```python
from build123d import *

# Parameters (mm, degrees)
SKETCH1_W           = 1700
SKETCH1_H           = 500
BOSS_EXTRUDE1_DEPTH = 5
SKETCH2_W           = 20
SKETCH2_H           = 20
BOSS_EXTRUDE2_DEPTH = 695
SKETCH3_W           = 900
SKETCH3_H           = 500
BOSS_EXTRUDE3_DEPTH = 30
SKETCH4_W           = 170
SKETCH4_H           = 500
CUT_EXTRUDE1_DEPTH  = 30


with BuildPart() as part:
    # Sketch1 → Boss-Extrude1 (new body)
    with BuildSketch(Plane(origin=(0, 0, 0), x_dir=(1, 0, 0), z_dir=(0, 1, 0))):
        with Locations((850, 250)):
            Rectangle(SKETCH1_W, SKETCH1_H)
    extrude(amount=BOSS_EXTRUDE1_DEPTH)

    # Sketch2 → Boss-Extrude2 (add)
    with BuildSketch(Plane(origin=(0, 5, 0), x_dir=(1, 0, 0), z_dir=(0, 1, 0))):
        with Locations((10, 490)):
            Rectangle(SKETCH2_W, SKETCH2_H)
        with Locations((10, 10)):
            Rectangle(SKETCH2_W, SKETCH2_H)
        with Locations((1690, 10)):
            Rectangle(SKETCH2_W, SKETCH2_H)
        with Locations((1690, 490)):
            Rectangle(SKETCH2_W, SKETCH2_H)
    extrude(amount=BOSS_EXTRUDE2_DEPTH)

    # Sketch3 → Boss-Extrude3 (add)
    with BuildSketch(Plane.XZ):
        with Locations((850, -250)):
            Rectangle(SKETCH3_W, SKETCH3_H)
    extrude(amount=BOSS_EXTRUDE3_DEPTH)

    # Sketch4 → Cut-Extrude1 (cut)
    with BuildSketch(Plane.XZ.offset(30)):
        with Locations((550, -250)):
            Rectangle(SKETCH4_W, SKETCH4_H)
        with Locations((850, -250)):
            Rectangle(SKETCH4_W, SKETCH4_H)
        with Locations((1150, -250)):
            Rectangle(SKETCH4_W, SKETCH4_H)
    extrude(amount=-CUT_EXTRUDE1_DEPTH, mode=Mode.SUBTRACT)


solid = part.part
```
Input: part model. Units: mm. Frame: model coordinates. A direction names the side the tool comes from. Coordinates: 2 decimals unless noted, no trailing zeros. Loops run counter-clockwise (first coordinate to the right, second up) from the corner with the lowest first, then second, coordinate; pieces in that order, holes last. Notation, with made-up numbers: (-36.5, 31.25) - (12.5, 31.25) arc R27 ccw to (12.5, 69.25) - close; hole circle Ø7 at (1.25, 87.5). An arc over 180 degrees is marked (long way). Answer in a Markdown table with one row per item.
(1) Material intervals for L1, parallel to Y at x = 838, z = -229.5; L2, parallel to Y at x = 637, z = -323.5, sorted ascending. Write a range as from..to.
Model answer:
| item | result |
|---|---|
| L1 | y = 0..5 |
| L2 | y = -30..5 |
(2) Mould query, pull axis X, two halves, no side actions, for faces 4 (the face through (699, -30, -246)), 5 (the face through (0, 348, -490)), 6 (the face through (549, 0, -246)). Classes: pulls with the +X half, pulls with the -X half, needs draft (parallel to the pull), parting line crosses it, or undercut.
Model answer:
| item | result |
|---|---|
| face 4 | needs draft |
| face 5 | pulls with the -X half |
| face 6 | undercut |
(3) Set-up query: faces 1 (the face through (1497, 0, -254)), 2 (the face through (465, -15, -253)), 3 (the face through (400, -15, -253)). Return all of +Z, -Z, +X, -X, +Y, -Y with unobstructed straight access to the full face (end or side cutting, diameter ignored); none if empty.
Model answer:
| item | result |
|---|---|
| face 1 | +Z, -Z, +X, -Y |
| face 2 | +Z, -Z, -Y |
| face 3 | +Z, -Z, -X, -Y |
(4) Pin query (flat end, axial travel): P1, Ø1, axis at x = 595.5, z = -184, coming from the -Y side; P2, Ø15, axis at y = -15.5, z = -231.5, coming from the +X side; P3, Ø15, axis at y = -11, z = -261.5, coming from the -X side. Return the tip coordinate at first contact, or that it passes through.
Model answer:
| item | result |
|---|---|
| P1 | stops at y = 0 |
| P2 | stops at x = 1300 |
| P3 | stops at x = 400 |
(5) Cut plane B-B on z = -359. Output: boundary loops of the cut face in (x, y), plus the area to 3 significant figures.
Model answer:
| item | result |
|---|---|
| outline | (0, 0) - (400, 0) - (400, -30) - (465, -30) - (465, 0) - (635, 0) - (635, -30) - (765, -30) - (765, 0) - (935, 0) - (935, -30) - (1065, -30) - (1065, 0) - (1235, 0) - (1235, -30) - (1300, -30) - (1300, 0) - (1700, 0) - (1700, 5) - (0, 5) - close |
| area | 20,200 mm² |
(6) Cut plane D-D on x = 1420. Output: boundary loops of the cut face in (y, z).
Model answer:
| item | result |
|---|---|
| outline | (0, -500) - (5, -500) - (5, 0) - (0, 0) - close |
(7) Cut plane C-C on x = 668.5. Output: boundary loops of the cut face in (y, z).
Model answer:
| item | result |
|---|---|
| outline | (-30, -500) - (5, -500) - (5, 0) - (-30, 0) - close |
(8) Cut plane A-A on y = 522. Output: boundary loops of the cut face in (x, z).
Model answer:
| item | result |
|---|---|
| outline | (0, -500) - (20, -500) - (20, -480) - (0, -480) - close; (0, -20) - (20, -20) - (20, 0) - (0, 0) - close; (1680, -500) - (1700, -500) - (1700, -480) - (1680, -480) - close; (1680, -20) - (1700, -20) - (1700, 0) - (1680, 0) - close |
